from build123d import *

# Parameters (mm, degrees)
SKETCH_3_W          = 80
SKETCH_3_H          = 50
EXTRUDE_3_DEPTH     = 8
SKETCH_4_W          = 80
SKETCH_4_H          = 86
EXTRUDE_4_DEPTH     = 8
SKETCH_7_W          = 100
SKETCH_7_H          = 18
CUT_EXTRUDE_1_DEPTH = 95
CUT_EXTRUDE_2_DEPTH = 87
SKETCH_9_R          = 11
CUT_EXTRUDE_3_DEPTH = 104.730419839
SKETCH_10_R         = 1.75
CUT_EXTRUDE_4_DEPTH = 104.730419839
EXTRUDE_7_DEPTH     = 6
EXTRUDE_8_DEPTH     = 6


with BuildPart() as part:
    # 草图3 → 凸台-拉伸3 (new body)
    with BuildSketch(Plane(origin=(0, 0, 0), x_dir=(1, 0, 0), z_dir=(0, 1, 0))):
        with Locations((0, -17)):
            Rectangle(SKETCH_3_W, SKETCH_3_H)
    extrude(amount=EXTRUDE_3_DEPTH)

    # 草图4 → 凸台-拉伸4 (add)
    with BuildSketch(Plane.XY):
        with Locations((0, 51)):
            Rectangle(SKETCH_4_W, SKETCH_4_H)
    extrude(amount=-EXTRUDE_4_DEPTH)

    # 草图7 → 切除-拉伸1 (cut, symmetric)
    with BuildSketch(Plane.XY):
        with Locations((0, 95)):
            Rectangle(SKETCH_7_W, SKETCH_7_H)
    extrude(amount=CUT_EXTRUDE_1_DEPTH, both=True, mode=Mode.SUBTRACT)

    # 草图8 → 切除-拉伸2 (cut, symmetric)
    with BuildSketch(Plane(origin=(0, 8, 0), x_dir=(1, 0, 0), z_dir=(0, 1, 0))):
        with BuildLine():
            Line((-22, -17), (-22, -31))
            ThreePointArc((-22, -31), (-25, -34), (-28, -31))
            Line((-28, -31), (-28, -17))
            ThreePointArc((-28, -17), (-25, -14), (-22, -17))
        make_face()
        with BuildLine():
            Line((28, -17), (28, -31))
            ThreePointArc((28, -31), (25, -34), (22, -31))
            Line((22, -31), (22, -17))
            ThreePointArc((22, -17), (25, -14), (28, -17))
        make_face()
    extrude(amount=CUT_EXTRUDE_2_DEPTH, both=True, mode=Mode.SUBTRACT)

    # 草图9 → 切除-拉伸3 (cut, through all)
    with BuildSketch(Plane.XY):
        with Locations((0, 52)):
            Circle(SKETCH_9_R)
    extrude(amount=-CUT_EXTRUDE_3_DEPTH, mode=Mode.SUBTRACT)

    # 草图10 → 切除-拉伸4 (cut, through all)
    with BuildSketch(Plane.XY):
        with Locations((-15.5, 67.5)):
            Circle(SKETCH_10_R)
        with Locations((15.5, 67.5)):
            Circle(SKETCH_10_R)
        with Locations((-15.5, 36.5)):
            Circle(SKETCH_10_R)
        with Locations((15.5, 36.5)):
            Circle(SKETCH_10_R)
    extrude(amount=-CUT_EXTRUDE_4_DEPTH, mode=Mode.SUBTRACT)

    # 草图11 → 凸台-拉伸7 (add)
    with BuildSketch(Plane(origin=(-40, 0, 0), x_dir=(0, 0, -1), z_dir=(1, 0, 0))):
        Polygon((0, 8), (-32, 8), (0, 40), align=None)
    extrude(amount=EXTRUDE_7_DEPTH)

    # 草图12 → 凸台-拉伸8 (add)
    with BuildSketch(Plane(origin=(34, 0, 0), x_dir=(0, 0, -1), z_dir=(1, 0, 0))):
        Polygon((0, 8), (-32, 8), (0, 40), align=None)
    extrude(amount=EXTRUDE_8_DEPTH)


solid = part.part
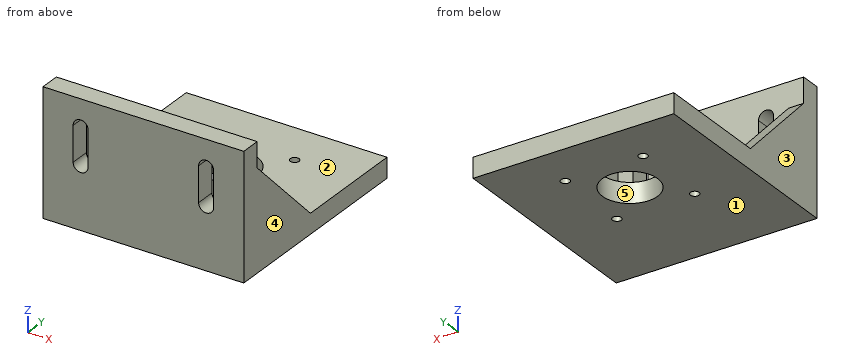
Design review of the part built by this model. Coordinates are the model's own, in mm. Face numbers are marked on the shaded views. A direction names the side the tool comes from. Give positions to 0.01 mm unless a question says otherwise; leave off trailing zeros. Order: outer loops, then holes, each group sorted by start corner. A loop starts at its lowest first (then second) coordinate and runs counter-clockwise, first axis right, second up.
1. Tool access review of the marked faces 1 and 2: name each direction out of +Z, -Z, +X, -X, +Y, -Y from which nothing blocks a thin tool from reaching the whole face with its end or side.
Solution:
face 1: -Z, +X, -X, +Y, -Y
face 2: +Z, +Y
2. Add section A-A, the plane y = 67.5. State the section outline as (x, z) points, then the cut area to 3 significant figures.
Solution:
outline: (-40, -8) - (-17.25, -8) - (-17.25, 0) - (-40, 0) - close; (-13.75, -8) - (13.75, -8) - (13.75, 0) - (-13.75, 0) - close; (17.25, -8) - (40, -8) - (40, 0) - (17.25, 0) - close
area: 584 mm2
3. For pin 1 Ø1 at (x, y) = (-21.5, 53) entering from +Z; pin 2 Ø8 at (x, y) = (-31, 42) entering from +Z; pin 3 Ø2 at (x, z) = (-10.5, 33) entering from +Y; pin 4 Ø2 at (x, y) = (15.5, 67.5) entering from +Z, all flat-tipped, find the tip position at first contact; note any pin that passes through.
Solution:
pin 1: stops at z = 0
pin 2: stops at z = 0.65
pin 3: stops at y = 8
pin 4: passes through
4. To check wall thickness, follow L1, parallel to Y at x = 15.5, z = -2.5; L2, parallel to X at y = 67.5, z = -1.25; L3, parallel to Y at x = 0, z = -4. State the ranges of each line that lie inside material, in increasing order.
Solution:
L1: y = 0 to 34.75, 38.25 to 65.75, 69.25 to 86
L2: x = -40 to -17.25, -13.75 to 13.75, 17.25 to 40
L3: y = 0 to 41, 63 to 86
5. Add section C-C, the plane z = -4. State the section outline as (x, y) points, then the cut area to 3 significant figures.
Solution:
outline: (-40, 0) - (40, 0) - (40, 86) - (-40, 86) - close; hole circle Ø3.5 at (-15.5, 36.5); hole circle Ø3.5 at (-15.5, 67.5); hole circle Ø22 at (0, 52); hole circle Ø3.5 at (15.5, 36.5); hole circle Ø3.5 at (15.5, 67.5)
area: 6,460 mm2
6. Mouldability with a two-part tool opening along X and no side actions: class the marked faces 3, 4 and 5 as +X half, -X half, draft (parallel to the pull), parting line (faces both ways), or undercut.
Solution:
face 3: -X half
face 4: +X half
face 5: undercut
7. Add section D-D, the plane x = -15.5. State the section outline as (y, z) points.
Solution:
outline: (0, -8) - (34.75, -8) - (34.75, 0) - (8, 0) - (8, 42) - (0, 42) - close; (38.25, -8) - (65.75, -8) - (65.75, 0) - (38.25, 0) - close; (69.25, -8) - (86, -8) - (86, 0) - (69.25, 0) - close
8. Add section B-B, the plane x = -25. State the section outline as (y, z) points, then the cut area to 3 significant figures.
Solution:
outline: (0, -8) - (86, -8) - (86, 0) - (8, 0) - (8, 14) - (0, 14) - close; (0, 34) - (8, 34) - (8, 42) - (0, 42) - close
area: 864 mm2
